Read the model definition and answer for the solid it produces. Units are mm, in the model's axes. Face numbers are marked on the shaded views. A direction names the side the tool comes from. Round coordinates to 2 decimals unless told otherwise and drop trailing zeros. Order: outer loops, then holes, each group sorted by start corner. A loop starts at its lowest first (then second) coordinate and runs counter-clockwise, first axis right, second up. Notation, with made-up numbers: M 38,-33 L 89,-33 A22 cw 89,-26 Z; hole C 38,-27.5 d9. An arc over 180 degrees is marked long. Answer as CSV lines item,"result".
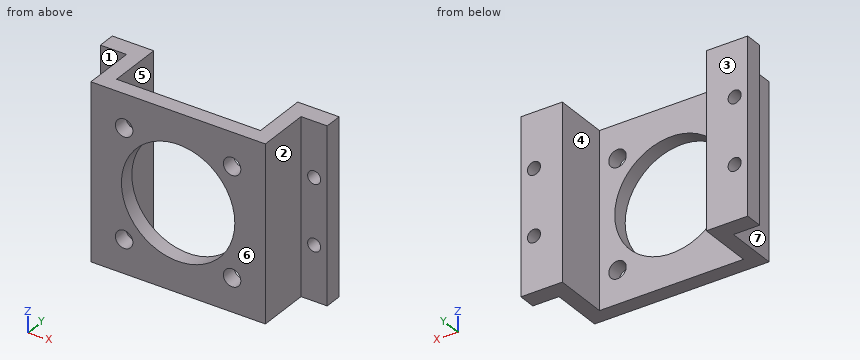
```python
from build123d import *

# Parameters (mm, degrees)
EXTRUDE_1_DEPTH          = 40
SKETCH_2_R               = 13
CUT_EXTRUDE_1_DEPTH      = 1.5
SKETCH_3_R               = 13
CUT_EXTRUDE_2_DEPTH      = 15.5
SKETCH_4_R               = 2
CUT_EXTRUDE_3_DEPTH      = 5
PATTERN_CIRCULAR_1_COUNT = 4
SKETCH_5_R               = 1.5
CUT_EXTRUDE_4_DEPTH      = 7
SKETCH_6_W               = 33
SKETCH_6_H               = 40
CUT_EXTRUDE_5_DEPTH      = 1.5
SKETCH_7_W               = 6
SKETCH_7_H               = 40
CUT_EXTRUDE_6_DEPTH      = 2


with BuildPart() as part:
    # 草图1 → 凸台-拉伸1 (new body)
    with BuildSketch(Plane.XY):
        Polygon((-16.5, 27.398785639), (-16.5, 16.398785639), (16.5, 16.398785639), (16.5, 27.398785639), (26, 27.398785639), (26, 21.398785639), (20, 21.398785639), (20, 16.398785639), (20, 11.398785639), (-20, 11.398785639), (-20, 21.398785639), (-26, 21.398785639), (-26, 27.398785639), align=None)
    extrude(amount=EXTRUDE_1_DEPTH)

    # 草图2 → 切除-拉伸1 (cut)
    with BuildSketch(Plane.XZ.offset(-11.398785639)):
        with Locations((0, 20)):
            Circle(SKETCH_2_R)
    extrude(amount=-CUT_EXTRUDE_1_DEPTH, mode=Mode.SUBTRACT)

    # 草图3 → 切除-拉伸2 (cut, through all)
    with BuildSketch(Plane.XZ.offset(-12.898785639)):
        with Locations((0, 20)):
            Circle(SKETCH_3_R)
    extrude(amount=-CUT_EXTRUDE_2_DEPTH, mode=Mode.SUBTRACT)

    # 草图4 → 切除-拉伸3 (cut)
    with BuildSketch(Plane.XZ.offset(-11.398785639)):
        with Locations((12.374368671, 32.374368671)):
            Circle(SKETCH_4_R)
    cut_extrude_3 = extrude(amount=-CUT_EXTRUDE_3_DEPTH, mode=Mode.SUBTRACT)

    # 阵列(圆周)1: 切除-拉伸3 ×4 about axis
    pattern_circular_1_axis = Axis((0, 0, 20), (0, 1, 0))
    for i in range(1, PATTERN_CIRCULAR_1_COUNT):
        add(cut_extrude_3.rotate(pattern_circular_1_axis, i * 360 / PATTERN_CIRCULAR_1_COUNT), mode=Mode.SUBTRACT)

    # 草图5 → 切除-拉伸4 (cut, through all)
    with BuildSketch(Plane.XZ.offset(-21.398785639)):
        with Locations((-23, 27.5)):
            Circle(SKETCH_5_R)
        with Locations((-23, 12.5)):
            Circle(SKETCH_5_R)
    cut_extrude_4 = extrude(amount=-CUT_EXTRUDE_4_DEPTH, mode=Mode.SUBTRACT)

    # 镜向1: 切除-拉伸4 across plane
    add(cut_extrude_4.mirror(Plane.ZY), mode=Mode.SUBTRACT)

    # 草图6 → 切除-拉伸5 (cut)
    with BuildSketch(Plane(origin=(0, 16.398785639, 0), x_dir=(1, 0, 0), z_dir=(0, 1, 0))):
        with Locations((0, -20)):
            Rectangle(SKETCH_6_W, SKETCH_6_H)
    extrude(amount=-CUT_EXTRUDE_5_DEPTH, mode=Mode.SUBTRACT)

    # 草图7 → 切除-拉伸6 (cut)
    with BuildSketch(Plane.XZ.offset(-21.398785639)):
        with Locations((-23, 20)):
            Rectangle(SKETCH_7_W, SKETCH_7_H)
        with Locations((23, 20)):
            Rectangle(SKETCH_7_W, SKETCH_7_H)
    extrude(amount=-CUT_EXTRUDE_6_DEPTH, mode=Mode.SUBTRACT)


solid = part.part
```
Item 1: A tool of negligible diameter and unlimited length cuts with its end or side. For the marked faces 1, 2, 3 and 4, from which of +Z, -Z, +X, -X, +Y, -Y can it reach the whole face along a straight path? Write none if from no direction.
Ans:
face 1,"+Z, -Z, -X, -Y"
face 2,"+Z, -Z, +X, -Y"
face 3,"+Z, -Z, +X, -X, +Y"
face 4,"+Z, -Z, +Y"
Item 2: A cutting plane is placed at A-A, the plane z = 20. Determine the outline of the cut face in (x, y).
Ans:
outline,"M -26,23.4 L -20,23.4 L -20,11.4 L -13,11.4 L -13,14.9 L -16.5,14.9 L -16.5,27.4 L -26,27.4 Z; M 13,11.4 L 20,11.4 L 20,23.4 L 26,23.4 L 26,27.4 L 16.5,27.4 L 16.5,14.9 L 13,14.9 Z"
Item 3: Find the intervals of material crossed by probe 1 along Z at (x, y) = (-23, 25); probe 2 along X at (y, z) = (22.25, 6.5); probe 3 along X at (y, z) = (24.75, 27), in increasing order. Write a range as [from, to].
Ans:
probe 1,"[0, 11], [14, 26], [29, 40]"
probe 2,"[-20, -16.5], [16.5, 20]"
probe 3,"[-26, -24.41], [-21.59, -16.5], [16.5, 21.59], [24.41, 26]"
Item 4: A cutting plane is placed at B-B, the plane y = 18.5. Determine the outline of the cut face in (x, z), and give its area (3 significant figures).
Ans:
outline,"M -20,0 L -16.5,0 L -16.5,40 L -20,40 Z; M 16.5,0 L 20,0 L 20,40 L 16.5,40 Z"
area,"280 mm2"
Item 5: A cutting plane is placed at D-D, the plane x = 0. Determine the outline of the cut face in (y, z).
Ans:
outline,"M 11.4,0 L 14.9,0 L 14.9,7 L 11.4,7 Z; M 11.4,33 L 14.9,33 L 14.9,40 L 11.4,40 Z"
Item 6: Flat-ended cylindrical pins translate along their axes: pin 1 (8 mm diameter, centred on y = 14, z = 35.5, fed in from +X); pin 2 (3.5 mm diameter, centred on x = -23, z = 12.5, fed in from -Y); pin 3 (6.5 mm diameter, centred on x = -12.37, z = 7.63, fed in from +Y). Find the tip coordinate at first contact, or state that the pin passes through.
Ans:
pin 1,"x = 20"
pin 2,"y = 23.4"
pin 3,"y = 14.9"
Item 7: Determine the mould class of the marked faces 5, 6 and 7 for opening direction X: +X half, -X half, draft (parallel to the pull), parting line (faces both ways), or undercut.
Ans:
face 5,"undercut"
face 6,"draft"
face 7,"-X half"
Item 8: A cutting plane is placed at C-C, the plane x = -23. Determine the outline of the cut face in (y, z), and give its area (3 significant figures).
Ans:
outline,"M 23.4,0 L 27.4,0 L 27.4,11 L 23.4,11 Z; M 23.4,14 L 27.4,14 L 27.4,26 L 23.4,26 Z; M 23.4,29 L 27.4,29 L 27.4,40 L 23.4,40 Z"
area,"136 mm2"
